from build123d import *

# Parameters (mm, degrees)
SKETCH1_W           = 76
SKETCH1_H           = 40
SKETCH1_R           = 2.6
BOSS_EXTRUDE1_DEPTH = 4
SKETCH2_W           = 15
SKETCH2_H           = 40
SKETCH2_R           = 2.6
BOSS_EXTRUDE2_DEPTH = 5.5
SKETCH3_R           = 4
SKETCH3_R_2         = 2.6
BOSS_EXTRUDE3_DEPTH = 2
CHAMFER1_SIZE       = 2
FILLET1_R           = 4


with BuildPart() as part:
    # Sketch1 → Boss-Extrude1 (new body)
    with BuildSketch(Plane(origin=(0, 0, 0), x_dir=(1, 0, 0), z_dir=(0, 1, 0))):
        Rectangle(SKETCH1_W, SKETCH1_H)
        with Locations(Location((-31, -13, 0), (0, 0, 270))):
            Circle(SKETCH1_R, mode=Mode.SUBTRACT)
        with Locations(Location((-31, 13, 0), (0, 0, 270))):
            Circle(SKETCH1_R, mode=Mode.SUBTRACT)
        with BuildLine():
            Line((30, 15.6), (32, 15.6))
            ThreePointArc((32, 15.6), (34.6, 13), (32, 10.4))
            Line((32, 10.4), (30, 10.4))
            ThreePointArc((30, 10.4), (27.4, 13), (30, 15.6))
        make_face(mode=Mode.SUBTRACT)
        with BuildLine():
            Line((32, -10.4), (30, -10.4))
            ThreePointArc((30, -10.4), (27.4, -13), (30, -15.6))
            Line((30, -15.6), (32, -15.6))
            ThreePointArc((32, -15.6), (34.6, -13), (32, -10.4))
        make_face(mode=Mode.SUBTRACT)
    extrude(amount=BOSS_EXTRUDE1_DEPTH)

    # Sketch2 → Boss-Extrude2 (add)
    # profile 1 of 2: a face of its own
    with BuildSketch(Plane(origin=(0, 4, 0), x_dir=(1, 0, 0), z_dir=(0, 1, 0))):
        with Locations((30.5, 0)):
            Rectangle(SKETCH2_W, SKETCH2_H)
        with BuildLine():
            ThreePointArc((30, -15.6), (27.4, -13), (30, -10.4))
            Line((30, -10.4), (32, -10.4))
            ThreePointArc((32, -10.4), (34.6, -13), (32, -15.6))
            Line((32, -15.6), (30, -15.6))
        make_face(mode=Mode.SUBTRACT)
        with BuildLine():
            ThreePointArc((30, 10.4), (27.4, 13), (30, 15.6))
            Line((30, 15.6), (32, 15.6))
            ThreePointArc((32, 15.6), (34.6, 13), (32, 10.4))
            Line((32, 10.4), (30, 10.4))
        make_face(mode=Mode.SUBTRACT)
    # profile 2 of 2: a face of its own
    with BuildSketch(Plane(origin=(0, 4, 0), x_dir=(1, 0, 0), z_dir=(0, 1, 0))):
        with Locations((-30.5, 0)):
            Rectangle(SKETCH2_W, SKETCH2_H)
        with Locations((-31, -13)):
            Circle(SKETCH2_R, mode=Mode.SUBTRACT)
        with Locations((-31, 13)):
            Circle(SKETCH2_R, mode=Mode.SUBTRACT)
    extrude(amount=BOSS_EXTRUDE2_DEPTH)

    # Sketch3 → Boss-Extrude3 (add)
    # profile 1 of 4: a face of its own
    with BuildSketch(Plane(origin=(0, 9.5, 0), x_dir=(1, 0, 0), z_dir=(0, 1, 0))):
        with Locations(Location((-31, 13, 0), (0, 0, 270))):
            Circle(SKETCH3_R)
        with Locations(Location((-31, 13, 0), (0, 0, 270))):
            Circle(SKETCH3_R_2, mode=Mode.SUBTRACT)
    # profile 2 of 4: a face of its own
    with BuildSketch(Plane(origin=(0, 9.5, 0), x_dir=(1, 0, 0), z_dir=(0, 1, 0))):
        with Locations(Location((-31, -13, 0), (0, 0, 270))):
            Circle(SKETCH3_R)
        with Locations(Location((-31, -13, 0), (0, 0, 270))):
            Circle(SKETCH3_R_2, mode=Mode.SUBTRACT)
    # profile 3 of 4: a face of its own
    with BuildSketch(Plane(origin=(0, 9.5, 0), x_dir=(1, 0, 0), z_dir=(0, 1, 0))):
        with BuildLine():
            Line((32, 17), (30, 17))
            ThreePointArc((30, 17), (26, 13), (30, 9))
            Line((30, 9), (32, 9))
            ThreePointArc((32, 9), (36, 13), (32, 17))
        make_face()
        with BuildLine():
            Line((30, 15.6), (32, 15.6))
            ThreePointArc((32, 15.6), (34.6, 13), (32, 10.4))
            Line((32, 10.4), (30, 10.4))
            ThreePointArc((30, 10.4), (27.4, 13), (30, 15.6))
        make_face(mode=Mode.SUBTRACT)
    # profile 4 of 4: a face of its own
    with BuildSketch(Plane(origin=(0, 9.5, 0), x_dir=(1, 0, 0), z_dir=(0, 1, 0))):
        with BuildLine():
            Line((32, -9), (30, -9))
            ThreePointArc((30, -9), (26, -13), (30, -17))
            Line((30, -17), (32, -17))
            ThreePointArc((32, -17), (36, -13), (32, -9))
        make_face()
        with BuildLine():
            Line((32, -10.4), (30, -10.4))
            ThreePointArc((30, -10.4), (27.4, -13), (30, -15.6))
            Line((30, -15.6), (32, -15.6))
            ThreePointArc((32, -15.6), (34.6, -13), (32, -10.4))
        make_face(mode=Mode.SUBTRACT)
    extrude(amount=BOSS_EXTRUDE3_DEPTH)

    # Chamfer1
    chamfer1_edges = [part.edges().sort_by_distance(p)[0] for p in [
        (-31, 9.5, 9),
        (-31, 9.5, -17),
        (31, 9.5, -17),
        (26, 9.5, -13),
        (31, 9.5, -9),
        (36, 9.5, -13),
        (31, 9.5, 9),
        (26, 9.5, 13),
        (36, 9.5, 13),
        (31, 9.5, 17),
    ]]
    chamfer(chamfer1_edges, length=CHAMFER1_SIZE - 0.0001)  # a hair under: the kernel refuses the full size

    # Fillet1
    fillet1_edges = [part.edges().sort_by_distance(p)[0] for p in [
        (38, 4.75, 20),
        (-38, 4.75, 20),
        (-38, 4.75, -20),
        (38, 4.75, -20),
        (-23, 6.75, 20),
        (-23, 6.75, -20),
        (23, 6.75, -20),
        (23, 6.75, 20),
    ]]
    fillet(fillet1_edges, radius=FILLET1_R)


solid = part.part
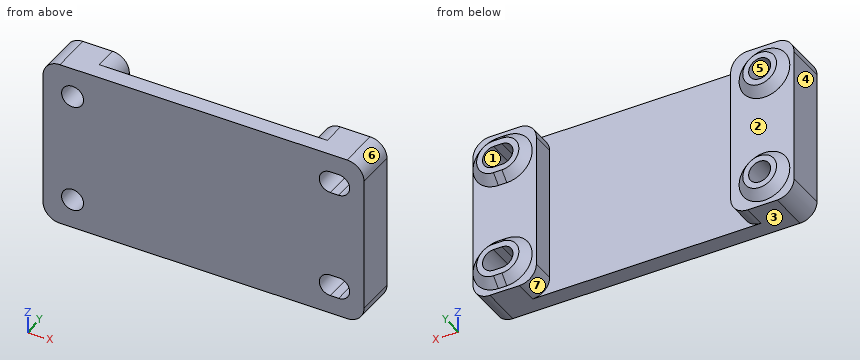
Verification items for the finished model (mm, model axes). Face numbers are marked on the shaded views. A direction names the side the tool comes from. Give positions to 0.01 mm unless a question says otherwise; leave off trailing zeros. Loops run counter-clockwise (first coordinate to the right, second up) from the corner with the lowest first, then second, coordinate; pieces in that order, holes last.
1. Cross-section at A-A on y = 5.25. Record the cut outline in (x, z), and give its area (3 significant figures).
Derived:
outline: (-38, -16) arc R4 ccw to (-34, -20) - (-27, -20) arc R4 ccw to (-23, -16) - (-23, 16) arc R4 ccw to (-27, 20) - (-34, 20) arc R4 ccw to (-38, 16) - close; (23, -16) arc R4 ccw to (27, -20) - (34, -20) arc R4 ccw to (38, -16) - (38, 16) arc R4 ccw to (34, 20) - (27, 20) arc R4 ccw to (23, 16) - close; hole circle Ø5.2 at (-31, -13); hole circle Ø5.2 at (-31, 13); hole (30, -15.6) - (32, -15.6) arc R2.6 ccw to (32, -10.4) - (30, -10.4) arc R2.6 ccw to start; hole (30, 10.4) - (32, 10.4) arc R2.6 ccw to (32, 15.6) - (30, 15.6) arc R2.6 ccw to start
area: 1,070 mm2
2. Cross-section at D-D on y = 1.5. Record the cut outline in (x, z).
Derived:
outline: (-38, -16) arc R4 ccw to (-34, -20) - (34, -20) arc R4 ccw to (38, -16) - (38, 16) arc R4 ccw to (34, 20) - (-34, 20) arc R4 ccw to (-38, 16) - close; hole circle Ø5.2 at (-31, -13); hole circle Ø5.2 at (-31, 13); hole (30, -15.6) - (32, -15.6) arc R2.6 ccw to (32, -10.4) - (30, -10.4) arc R2.6 ccw to start; hole (30, 10.4) - (32, 10.4) arc R2.6 ccw to (32, 15.6) - (30, 15.6) arc R2.6 ccw to start
3. Go/stop test with flat-tipped pins: P1, Ø3, axis at x = -31, z = -13, coming from the -Y side; P2, Ø4.5, axis at x = -29, z = -3, coming from the +Y side. Record where each tip stops, or that it passes through.
Derived:
P1: passes through
P2: stops at y = 9.5
4. Release check for a two-part mould opening along Z. For the marked faces 4, 5, 6 and 7 record: +Z half, -Z half, draft (parallel to the pull), parting line (faces both ways), or undercut.
Derived:
face 4: draft
face 5: undercut
face 6: +Z half
face 7: -Z half
5. Tool access check on the marked faces 1, 2 and 3. Record the directions out of +Z, -Z, +X, -X, +Y, -Y that give a thin tool (end or side, any length) a straight path to the whole face; none if there is none.
Derived:
face 1: +Y, -Y
face 2: +Y
face 3: -Z, +X, -X, +Y, -Y
6. Material ranges on probe 1 along X at (y, z) = (5.75, -13); probe 2 along X at (y, z) = (3.5, 13); probe 3 along X at (y, z) = (9, 11), recorded low to high.
Derived:
probe 1: x = -38 to -33.6, -28.4 to -23, 23 to 27.4, 34.6 to 38
probe 2: x = -38 to -33.6, -28.4 to 27.4, 34.6 to 38
probe 3: x = -38 to -32.66, -29.34 to -23, 23 to 28.34, 33.66 to 38
7. Cross-section at B-B on z = -13. Count the separate pieces of the cut face and the enclosed holes in it, and give its area (3 significant figures).
Derived:
separate pieces: 3
enclosed holes: 0
area: 370 mm2
